Geometry: final body of the model. Coordinates: model frame, mm. Round coordinates to 2 decimals unless told otherwise and drop trailing zeros. Loops run counter-clockwise (first coordinate to the right, second up) from the corner with the lowest first, then second, coordinate; pieces in that order, holes last. Notation, with made-up numbers: (61.5, 1.5) - (75.5, 1.5) arc R18 cw to (75.5, 18.5) - close; hole circle Ø4 at (19.25, 39). An arc over 180 degrees is marked (long way). Answer as a JSON object with one key per item and string values. Group by question number.
Item 1: Section B-B (z = -1075). Count the separate pieces of the cut face and the enclosed holes in it, plus the area to 3 significant figures.
Item 2: First-contact query: pin 1 (8 mm diameter, centred on x = 102.5, z = -415.5, fed in from -Y); pin 2 (8 mm diameter, centred on x = 502, z = -859.5, fed in from +Y). Flat tips, straight axial feed; report the tip coordinate or a pass-through.
Item 3: Section A-A (y = 8.5). Return the cut outline in (x, z), plus the area to 3 significant figures.
Item 4: Line query: line 1 (Z direction, x = 334, y = 64.5); line 2 (Y direction, x = 806.5, z = -218); line 3 (Y direction, x = 863, z = -818.5). Output: solid intervals per line, ascending.
```python
from build123d import *

# Parameters (mm, degrees)
SKETCH3_W           = 40
SKETCH3_H           = 30
SKETCH4_R           = 12.5
BOSS_EXTRUDE1_DEPTH = 1180
LPATTERN1_COUNT     = 10
LPATTERN1_PITCH     = 120
LPATTERN2_COUNT     = 2
LPATTERN2_PITCH     = 1180
SKETCH5_R           = 12.5
BOSS_EXTRUDE2_DEPTH = 1170
LPATTERN3_COUNT     = 10
LPATTERN3_PITCH     = 120


with BuildPart() as part:
    # Sweep1: sweep along a path in Sketch2
    with BuildLine(Plane.XY) as sweep1_path:
        Line((0, 50), (1200, 50))
        ThreePointArc((1200, 50), (1250, 0), (1200, -50))
        Line((1200, -50), (0, -50))
        ThreePointArc((0, -50), (-50, 0), (0, 50))
    # Sketch3 → Sweep1 (sweep)
    with BuildSketch(Plane(origin=(0, 0, 0), x_dir=(0, 0, -1), z_dir=(1, 0, 0))):
        with Locations((0, 58.363712196)):
            Rectangle(SKETCH3_W, SKETCH3_H)
    sweep1 = sweep(path=sweep1_path.line)

    # Sketch4 → Boss-Extrude1 (add)
    with BuildSketch(Plane(origin=(0, 0, -20), x_dir=(-1, 0, 0), z_dir=(0, 0, -1))):
        with Locations(Location((-1092.450954457, 58.961219157, 0), (0, 0, 270))):
            Circle(SKETCH4_R)
    boss_extrude1 = extrude(amount=BOSS_EXTRUDE1_DEPTH)

    # LPattern1: Boss-Extrude1 ×10
    with Locations(*[(-i * LPATTERN1_PITCH, 0, 0) for i in range(1, LPATTERN1_COUNT)]):
        add(boss_extrude1)

    # LPattern2: Sweep1 ×2
    with Locations(*[(0, 0, -i * LPATTERN2_PITCH) for i in range(1, LPATTERN2_COUNT)]):
        add(sweep1)

    # Sketch5 → Boss-Extrude2 (add)
    with BuildSketch(Plane(origin=(0, 0, -20), x_dir=(-1, 0, 0), z_dir=(0, 0, -1))):
        with Locations(Location((-1172.681087279, -60.134950417, 0), (0, 0, 270))):
            Circle(SKETCH5_R)
    boss_extrude2 = extrude(amount=BOSS_EXTRUDE2_DEPTH)

    # LPattern3: Boss-Extrude2 ×10
    with Locations(*[(-i * LPATTERN3_PITCH, 0, 0) for i in range(1, LPATTERN3_COUNT)]):
        add(boss_extrude2)


solid = part.part
```
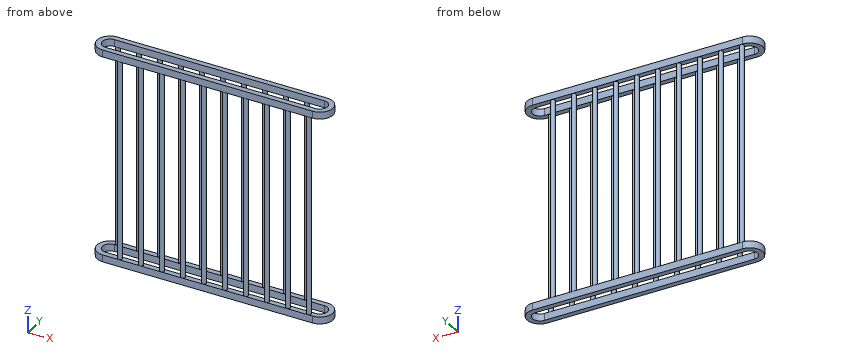
Values:
{
 "1": {"separate pieces": "20", "enclosed holes": "0", "area": "9,820 mm^2"},
 "2": {"pin 1": "stops at y = -71.2", "pin 2": "stops at y = 70.16"},
 "3": {"outline": "(-72.87, -1200) - (-42.52, -1200) - (-42.52, -1160) - (-72.87, -1160) - close; (-72.87, -20) - (-42.52, -20) - (-42.52, 20) - (-72.87, 20) - close; (1242.52, -1200) - (1272.87, -1200) - (1272.87, -1160) - (1242.52, -1160) - close; (1242.52, -20) - (1272.87, -20) - (1272.87, 20) - (1242.52, 20) - close", "area": "4,860 mm^2"},
 "4": {"line 1": "z = -1200 to -1160, -20 to 20", "line 2": "y = -71 to -49.27", "line 3": "y = 52.26 to 65.67"}
}
